```python
from build123d import *

# Parameters (mm, degrees)
SKETCH1_W           = 26
SKETCH1_H           = 11.5
BOSS_EXTRUDE1_DEPTH = 3
FILLET1_R           = 4
BOSS_EXTRUDE2_DEPTH = 3
FILLET2_R           = 4
BOSS_EXTRUDE3_DEPTH = 3
CUT_EXTRUDE2_DEPTH  = 4
FILLET3_R           = 4
SKETCH5_R           = 1.2
CUT_EXTRUDE3_DEPTH  = 4


with BuildPart() as part:
    # Sketch1 → Boss-Extrude1 (new body)
    with BuildSketch(Plane(origin=(0, 0, 0), x_dir=(1, 0, 0), z_dir=(0, 1, 0))):
        Rectangle(SKETCH1_W, SKETCH1_H)
    extrude(amount=BOSS_EXTRUDE1_DEPTH)

    # Fillet1
    fillet1_edges = [part.edges().sort_by_distance(p)[0] for p in [
        (13, 1.5, 5.75),
        (-13, 1.5, 5.75),
        (-13, 1.5, -5.75),
        (13, 1.5, -5.75),
    ]]
    fillet(fillet1_edges, radius=FILLET1_R)

    # Sketch2 → Boss-Extrude2 (add)
    with BuildSketch(Plane(origin=(1.8, 0, 0), x_dir=(0, 0, -1), z_dir=(1, 0, 0))):
        Polygon((0, 3), (5.75, 3), (5.75, -1.5), (16, -1.5), (16, 3), (16, 9.5), (0, 9.5), (-5.75, 9.5), (-5.75, 3), align=None)
    extrude(amount=BOSS_EXTRUDE2_DEPTH)

    # Fillet2
    fillet2_edges = [part.edges().sort_by_distance(p)[0] for p in [
        (3.3, 9.5, 5.75),
    ]]
    fillet(fillet2_edges, radius=FILLET2_R)

    # Sketch4 → Boss-Extrude3 (add)
    with BuildSketch(Plane.ZY.offset(-1.8)):
        with BuildLine():
            Line((-7.075, 9.5), (-7.075, -1.5))
            Line((-7.075, -1.5), (-5.75, -1.5))
            Line((-5.75, -1.5), (-5.75, 0))
            Line((-5.75, 0), (-5.75, 3))
            Line((-5.75, 3), (5.75, 3))
            Line((5.75, 3), (5.75, 5.5))
            ThreePointArc((5.75, 5.5), (4.578427125, 8.328427125), (1.75, 9.5))
            Line((1.75, 9.5), (-7.075, 9.5))
        make_face()
    extrude(amount=BOSS_EXTRUDE3_DEPTH)

    # Sketch3 → Cut-Extrude2 (cut)
    with BuildSketch(Plane(origin=(4.8, 0, 0), x_dir=(0, 0, -1), z_dir=(1, 0, 0))):
        with BuildLine():
            Line((9.75, 2.25), (9.75, 5.75))
            ThreePointArc((9.75, 5.75), (11, 7), (12.25, 5.75))
            Line((12.25, 5.75), (12.25, 2.25))
            ThreePointArc((12.25, 2.25), (11, 1), (9.75, 2.25))
        make_face()
    extrude(amount=-CUT_EXTRUDE2_DEPTH, mode=Mode.SUBTRACT)

    # Fillet3
    fillet3_edges = [part.edges().sort_by_distance(p)[0] for p in [
        (3.3, -1.5, -16),
        (3.3, 9.5, -16),
    ]]
    fillet(fillet3_edges, radius=FILLET3_R)

    # Sketch5 → Cut-Extrude3 (cut)
    with BuildSketch(Plane.XZ):
        with Locations(Location((8.997973452, -0.000616233, 0), (0, 0, 270))):
            Circle(SKETCH5_R)
        with Locations(Location((-9.000145119, 0.001069025, 0), (0, 0, 270))):
            Circle(SKETCH5_R)
    extrude(amount=-CUT_EXTRUDE3_DEPTH, mode=Mode.SUBTRACT)


solid = part.part
```
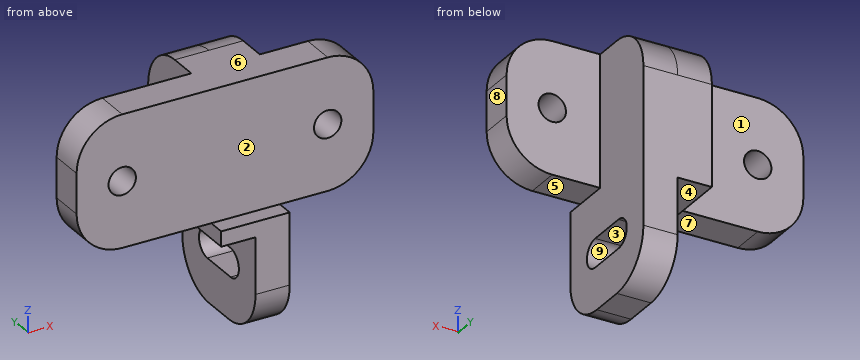
Design review of the part built by this model. Coordinates are the model's own, in mm. Face numbers are marked on the shaded views. A direction names the side the tool comes from. Coordinates: 2 decimals unless noted, no trailing zeros. Order: outer loops, then holes, each group sorted by start corner. A loop starts at its lowest first (then second) coordinate and runs counter-clockwise, first axis right, second up.
1) Mouldability with a two-part tool opening along Z and no side actions: class the marked faces 6, 7, 8 and 9 as +Z half, -Z half, draft (parallel to the pull), parting line (faces both ways), or undercut.
2) Clearance check with flat-ended pins moving along their axes: pin 1 (2 mm diameter, centred on x = -3, z = 1.5, fed in from +Y); pin 2 (2 mm diameter, centred on y = 0.5, z = -4.5, fed in from -X); pin 3 (6 mm diameter, centred on x = 3.5, z = -1, fed in from -Y). State where each tip first meets the part, or that it passes through.
3) Take a section at C-C, the plane x = -3. Give the boundary of the cut face in (y, z), and give its area (3 significant figures).
4) Take a section at A-A, the plane z = -11. Give the boundary of the cut face in (x, y).
5) Wall thickness on line 1 along Y through (x, z) = (0.25, 1.5); line 2 along Y through (x, z) = (-3, 1); line 3 along Z through (x, y) = (7, 1.75): over which ranges is each line inside the solid? List them lowest first.
6) Take a section at B-B, the plane z = -5.25. Give the boundary of the cut face in (x, y).
7) For the marked faces 1, 2, 3, 4 and 5, list the 3-axis set-ups (+Z, -Z, +X, -X, +Y, -Y) from which the entire face can be reached by the end or side of a thin tool; tool diameter is ignored.
Returned:
1. face 6: +Z half
1. face 7: -Z half
1. face 8: draft
1. face 9: undercut
2. pin 1: stops at y = 3
2. pin 2: stops at x = -12.6
2. pin 3: stops at y = 0
3. outline: (0, -5.75) - (3, -5.75) - (3, 5.75) - (0, 5.75) - close
3. area: 34.5 mm2
4. outline: (1.8, -1.5) - (4.8, -1.5) - (4.8, 1) - (1.8, 1) - close; (1.8, 7) - (4.8, 7) - (4.8, 9.5) - (1.8, 9.5) - close
5. line 1: y = 0 to 9.5
5. line 2: y = 0 to 3
5. line 3: z = -5.75 to 5.75
6. outline: (-10.94, 0) - (10.94, 0) - (10.94, 3) - (4.8, 3) - (4.8, 9.5) - (-1.2, 9.5) - (-1.2, 3) - (-10.94, 3) - close
7. face 1: +Z, -Z, -X, +Y
7. face 2: +Z, +X, -X, -Y
7. face 3: +X, -X
7. face 4: -Z, -X, +Y, -Y
7. face 5: -Z, +X, +Y, -Y
